For this review, use the dimensioned drawing (mm, ordinates from the lowest corner) and the shaded views. A direction names the side the tool comes from. Give positions to 0.01 mm unless a question says otherwise; leave off trailing zeros. Loops run counter-clockwise (first coordinate to the right, second up) from the corner with the lowest first, then second, coordinate; pieces in that order, holes last. Notation, with made-up numbers: M 28,-30.75 L 75,-30.75 A28 cw 75,4.25 Z; hole C 38.5,-37 d7. An arc over 180 degrees is marked long. Use CSV: the item, a comma, the result in double quotes. Start each with the question number.
1. Take a section at C-C, the plane z = 2.5. Write out the cut boundary in (x, y), and give its area (3 significant figures).
2. Tool access review of the marked faces 1 and 2: name each direction out of +Z, -Z, +X, -X, +Y, -Y from which nothing blocks a thin tool from reaching the whole face with its end or side.
3. Take a section at D-D, the plane x = 32. Write out the cut boundary in (y, z), and give its area (3 significant figures).
4. Insertion check: P1, Ø1.8, axis at y = 19.5, z = 4, coming from the +X side; P2, Ø3, axis at y = 51, z = 2, coming from the +X side; P3, Ø2, axis at y = 54.5, z = 2.5, coming from the +X side. Each pin has a flat end and moves straight along its axis. Give the tip position at first contact, or say it passes through.
5. The part is to be moulded in two halves that separate along Y. For the marked faces 3, 4 and 5, say which applies: pulls with the +Y half, pulls with the -Y half, needs draft (parallel to the pull), parting line crosses it, or undercut.
6. Take a section at A-A, the plane x = 9. Write out the cut boundary in (y, z), and give its area (3 significant figures).
7. To check wall thickness, follow line 1 (Y direction, x = 13, z = 1.85); line 2 (Y direction, x = 9.5, z = 4.55); line 3 (X direction, y = 40.5, z = 3.4). State the ranges of each line that lie inside material, in increasing order. Write a range as [from, to].
8. Take a section at B-B, the plane y = 6. Write out the cut boundary in (x, z), and give its area (3 significant figures).
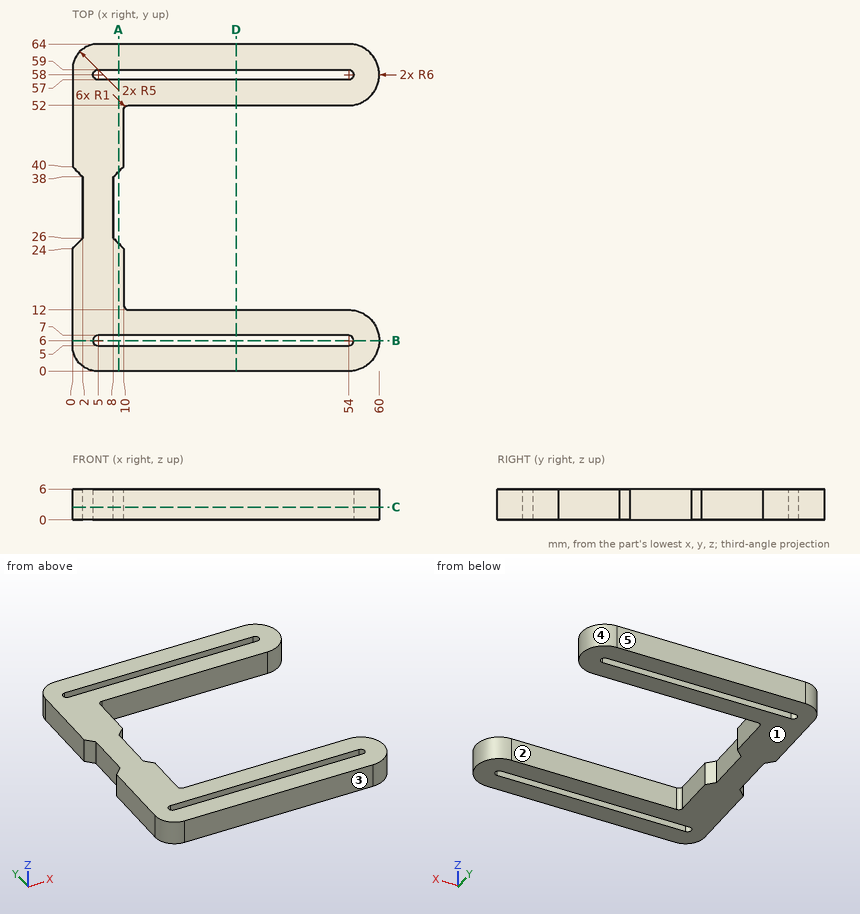
Result set:
1,outline,"M 0,5 A5 ccw 5,0 L 54,0 A6 ccw 54,12 L 11,12 A1 cw 10,13 L 10,24 L 8,26 L 8,38 L 10,40 L 10,51 A1 cw 11,52 L 54,52 A6 ccw 54,64 L 5,64 A5 ccw 0,59 L 0,40 L 2,38 L 2,26 L 0,24 Z; hole M 5,5 L 54,5 A1 ccw 54,7 L 5,7 A1 ccw Z; hole M 5,57 L 54,57 A1 ccw 54,59 L 5,59 A1 ccw Z"
1,area,"1,540 mm2"
2,face 1,"-Z, +X, -X, +Y, -Y"
2,face 2,"+Z, -Z, +X"
3,outline,"M 0,0 L 5,0 L 5,6 L 0,6 Z; M 7,0 L 12,0 L 12,6 L 7,6 Z; M 52,0 L 57,0 L 57,6 L 52,6 Z; M 59,0 L 64,0 L 64,6 L 59,6 Z"
3,area,"120 mm2"
4,P1,"x = 10"
4,P2,"x = 56.4"
4,P3,"x = 59.45"
5,face 3,"pulls with the -Y half"
5,face 4,"undercut"
5,face 5,"pulls with the +Y half"
6,outline,"M 0,0 L 5,0 L 5,6 L 0,6 Z; M 7,0 L 25,0 L 25,6 L 7,6 Z; M 39,0 L 57,0 L 57,6 L 39,6 Z; M 59,0 L 64,0 L 64,6 L 59,6 Z"
6,area,"276 mm2"
7,line 1,"[0, 5], [7, 12], [52, 57], [59, 64]"
7,line 2,"[0, 5], [7, 24.5], [39.5, 57], [59, 64]"
7,line 3,"[0, 10]"
8,outline,"M 0,0 L 4,0 L 4,6 L 0,6 Z; M 55,0 L 60,0 L 60,6 L 55,6 Z"
8,area,"54.0 mm2"
